Check sheet for the modelled part. Datum: model origin and axes. Units: mm. Give positions to 0.01 mm unless a question says otherwise; leave off trailing zeros. Order: outer loops, then holes, each group sorted by start corner. A loop starts at its lowest first (then second) coordinate and runs counter-clockwise, first axis right, second up. Notation, with made-up numbers: (34, -21) -> (49, -21) arc R14 cw to (49, -16) -> close; hole circle Ø11 at (12.25, 63). An arc over 180 degrees is marked (long way). Answer in a Markdown table with one row per item. Add a question column.
(1) Cross-section at C-C (x = 16). Record the cut outline in (y, z), then the cut area to 3 significant figures.
(2) Cross-section at D-D (z = 16). Record the cut outline in (x, y), then the cut area to 3 significant figures.
(3) Go/stop test with flat-tipped pins: pin 1 (2.5 mm diameter, centred on x = 0, z = 8, fed in from +Y); pin 2 (3 mm diameter, centred on x = 14.5, y = 1.5, fed in from +Z); pin 3 (2 mm diameter, centred on x = -13.5, y = 4, fed in from -Z); pin 4 (1.5 mm diameter, centred on x = -19, y = 3, fed in from +Z). Record where each tip stops, or that it passes through.
(4) Thickness scan on L1, parallel to X at y = 5, z = 8; L2, parallel to X at y = 2, z = 3; L3, parallel to Z at x = 16.5, y = 5. Record the ranges inside material, lowest first. Write a range as [from, to].
(5) Cross-section at A-A (z = 0). State how many separate pieces and enclosed holes the cut face has, then the cut area to 3 significant figures.
(6) Release check for a two-part mould opening along Z. For faces 1 (the face through (-6.309, 3.944, 28.413)), 2 (the face through (1.13, 4.06, 22.23)), 3 (the face through (6, 0, 6)) record: released by +Z, released by -Z, zero draft, split by the parting line, or undercut.
```python
from build123d import *

# Parameters (mm, degrees)
SKETCH_1_R          = 29.105
EXTRUDE_1_DEPTH     = 8
SKETCH_2_R          = 4
CUT_EXTRUDE_1_DEPTH = 8
SKETCH_3_R          = 2.1
CUT_EXTRUDE_2_DEPTH = 8


with BuildPart() as part:
    # 스케치1 → 보스-돌출1 (new body)
    with BuildSketch(Plane(origin=(0, 0, 0), x_dir=(1, 0, 0), z_dir=(0, 1, 0))):
        Circle(SKETCH_1_R)
    extrude(amount=EXTRUDE_1_DEPTH)

    # 스케치2 → 컷-돌출1 (cut)
    with BuildSketch(Plane(origin=(0, 8, 0), x_dir=(1, 0, 0), z_dir=(0, 1, 0))):
        Circle(SKETCH_2_R)
    extrude(amount=-CUT_EXTRUDE_1_DEPTH, mode=Mode.SUBTRACT)

    # 스케치3 → 컷-돌출2 (cut)
    with BuildSketch(Plane(origin=(0, 8, 0), x_dir=(1, 0, 0), z_dir=(0, 1, 0))):
        with Locations((0, 8)):
            Circle(SKETCH_3_R)
        with Locations((0, 16)):
            Circle(SKETCH_3_R)
        with Locations((0, 24)):
            Circle(SKETCH_3_R)
        with Locations((-8, 0)):
            Circle(SKETCH_3_R)
        with Locations((-16, 0)):
            Circle(SKETCH_3_R)
        with Locations((-24, 0)):
            Circle(SKETCH_3_R)
        with Locations((0, -8)):
            Circle(SKETCH_3_R)
        with Locations((0, -16)):
            Circle(SKETCH_3_R)
        with Locations((0, -24)):
            Circle(SKETCH_3_R)
        with Locations((8, 0)):
            Circle(SKETCH_3_R)
        with Locations((16, 0)):
            Circle(SKETCH_3_R)
        with Locations((24, 0)):
            Circle(SKETCH_3_R)
    extrude(amount=-CUT_EXTRUDE_2_DEPTH, mode=Mode.SUBTRACT)


solid = part.part
```
Answer below:
| question | item | result |
|---|---|---|
| 1 | outline | (0, -24.31) -> (8, -24.31) -> (8, -2.1) -> (0, -2.1) -> close; (0, 2.1) -> (8, 2.1) -> (8, 24.31) -> (0, 24.31) -> close |
| 1 | area | 355 mm² |
| 2 | outline | (-24.31, 0) -> (-2.1, 0) -> (-2.1, 8) -> (-24.31, 8) -> close; (2.1, 0) -> (24.31, 0) -> (24.31, 8) -> (2.1, 8) -> close |
| 2 | area | 355 mm² |
| 3 | pin 1 | passes through |
| 3 | pin 2 | stops at z = 26.04 |
| 3 | pin 3 | stops at z = -26.28 |
| 3 | pin 4 | stops at z = 22.67 |
| 4 | L1 | x = [-27.98, -2.1], [2.1, 27.98] |
| 4 | L2 | x = [-28.95, -2.65], [2.65, 28.95] |
| 4 | L3 | z = [-23.98, -2.04], [2.04, 23.98] |
| 5 | separate pieces | 8 |
| 5 | enclosed holes | 0 |
| 5 | area | 200 mm² |
| 6 | face 1 | split by the parting line |
| 6 | face 2 | undercut |
| 6 | face 3 | zero draft |
